```python
from build123d import *

# Parameters (mm, degrees)
EXTRUSION1_DEPTH        = 6
ESQUISSE7_W             = 30
ESQUISSE7_H             = 1
ENL_V_MAT_EXTRU_1_DEPTH = 6


with BuildPart() as part:
    # Esquisse1 → Extrusion1 (new body)
    with BuildSketch(Plane(origin=(0, 0, 0), x_dir=(1, 0, 0), z_dir=(0, 1, 0))):
        with BuildLine():
            Line((-24.25, -7.25), (24.25, -7.25))
            ThreePointArc((24.25, -7.25), (25.664213562, -6.664213562), (26.25, -5.25))
            Line((26.25, -5.25), (26.25, 5.25))
            ThreePointArc((26.25, 5.25), (25.664213562, 6.664213562), (24.25, 7.25))
            Line((24.25, 7.25), (-24.25, 7.25))
            ThreePointArc((-24.25, 7.25), (-25.664213562, 6.664213562), (-26.25, 5.25))
            Line((-26.25, 5.25), (-26.25, -5.25))
            ThreePointArc((-26.25, -5.25), (-25.664213562, -6.664213562), (-24.25, -7.25))
        make_face()
    extrude(amount=EXTRUSION1_DEPTH)

    # Esquisse6 → Révolution1 (revolve)
    with BuildSketch(Plane.XY):
        Polygon((-12, 0), (-12, -5), (-13.75, -5), (-15, -3.5), (-14.5, -3.5), (-14.5, 0), align=None)
    r_volution1 = revolve(axis=Axis((-12, 10.671623644, 0), (0, -1, 0)))

    # Symétrie1: Révolution1 across plane
    add(r_volution1.mirror(Plane(origin=(0, 0, 0), x_dir=(0, 0, 1), z_dir=(1, 0, 0))))

    # Esquisse7 → Enlèv. mat.-Extru.1 (cut, through all)
    with BuildSketch(Plane.XZ):
        Rectangle(ESQUISSE7_W, ESQUISSE7_H)
    extrude(amount=ENL_V_MAT_EXTRU_1_DEPTH, mode=Mode.SUBTRACT)


solid = part.part
```
Work out the finished part from the listing and answer in its coordinate system (mm). A direction names the side the tool comes from. Give positions to 0.01 mm unless a question says otherwise; leave off trailing zeros. Write each loop counter-clockwise with the first axis right and the second up, starting at its lowest first coordinate (ties: lowest second). Pieces come first, ordered by that corner, then holes.
(1) Which of the six approach directions +Z, -Z, +X, -X, +Y, -Y give full straight-line access (tool end or side, diameter ignored) to faces 1 (the flat face through (12, -5, 1)), 2 (the flat face through (12, -2, 0.5)), 3 (the cylindrical face through (-12, -1.7, -2.5)), 4 (the cylindrical face through (-12, -1.7, 2.5))?
Final values:
face 1: +Z, -Z, +X, -X, -Y
face 2: +X, -X, -Y
face 3: -Z
face 4: +Z
(2) The part is cut by section C-C on x = 7. Write down the section's boundary in (y, z).
Final values:
outline: (0, -7.25) - (6, -7.25) - (6, 7.25) - (0, 7.25) - close
(3) The part is cut by section B-B on z = 4.5. Write down the section's boundary in (x, y).
Final values:
outline: (-26.25, 0) - (26.25, 0) - (26.25, 6) - (-26.25, 6) - close
(4) The part is cut by section A-A on y = -2. Write down the section's boundary in (x, z).
Final values:
outline: (-14.45, -0.5) arc R2.5 ccw to (-9.55, -0.5) - close; (-14.45, 0.5) - (-9.55, 0.5) arc R2.5 ccw to start; (9.55, -0.5) arc R2.5 ccw to (14.45, -0.5) - close; (9.55, 0.5) - (14.45, 0.5) arc R2.5 ccw to start
(5) Straight lines are drawn through the part: line 1 (Y direction, x = 5.5, z = 5.25); line 2 (Z direction, x = 10, y = -0.75); line 3 (X direction, y = -2, z = -1.75). For each, find the intervals that lie inside material, in ascending order.
Final values:
line 1: y = 0 to 6
line 2: z = -1.5 to -0.5, 0.5 to 1.5
line 3: x = -13.79 to -10.21, 10.21 to 13.79
(6) The mould has two halves that part along X. Classify faces 5 (the cylindrical face through (25.68, 2.96, -6.65)), 6 (the flat face through (-12, -2, -0.5)), 7 (the flat face through (-11.8, -3.5, -2.7)): pulls with the +X half, pulls with the -X half, needs draft (parallel to the pull), parting line crosses it, or undercut.
Final values:
face 5: pulls with the +X half
face 6: needs draft
face 7: undercut
(7) Flat-ended cylindrical pins translate along their axes: pin 1 Ø2.5 at (x, y) = (12.5, -3.5) entering from +Z; pin 2 Ø2.5 at (x, y) = (12, -3) entering from -Z. Find the tip coordinate at first contact, or state that the pin passes through.
Final values:
pin 1: stops at z = 3
pin 2: stops at z = -3
